Input: dimensioned drawing with shaded views. Units: mm. Origin: part minimum x, y, z. Round coordinates to 2 decimals unless told otherwise and drop trailing zeros. Loops run counter-clockwise (first coordinate to the right, second up) from the corner with the lowest first, then second, coordinate; pieces in that order, holes last.
Item 1: Section query B-B on x = 127. Return loops of the section in (y, z).
Item 2: Section query A-A on z = 101.6. Return loops of the section in (x, y).
Item 3: First-contact query: P1, Ø8, axis at x = 102, z = 48.5, coming from the -Y side; P2, Ø20.5, axis at x = 15.875, z = 57.15, coming from the -Y side. Flat tips, straight axial feed; report the tip coordinate or a pass-through.
Item 4: Section query D-D on y = 4.5. Return loops of the section in (x, z) (3 decimals), then the cut area to 3 significant figures.
Item 5: Section query C-C on z = 57.15. Return loops of the section in (x, y) (3 decimals).
Item 6: Pull-direction query (X, two-part tool) for the marked faces 1, 2 and 3; classes: released by +X, released by -X, zero draft, split by the parting line, or undercut.
Item 7: Ray query, L1, parallel to Z at x = 127, y = 3; L2, parallel to X at y = 6.25, z = 101.6; L3, parallel to X at y = 1.75, z = 57.5. Return the intervals inside material, ascending.
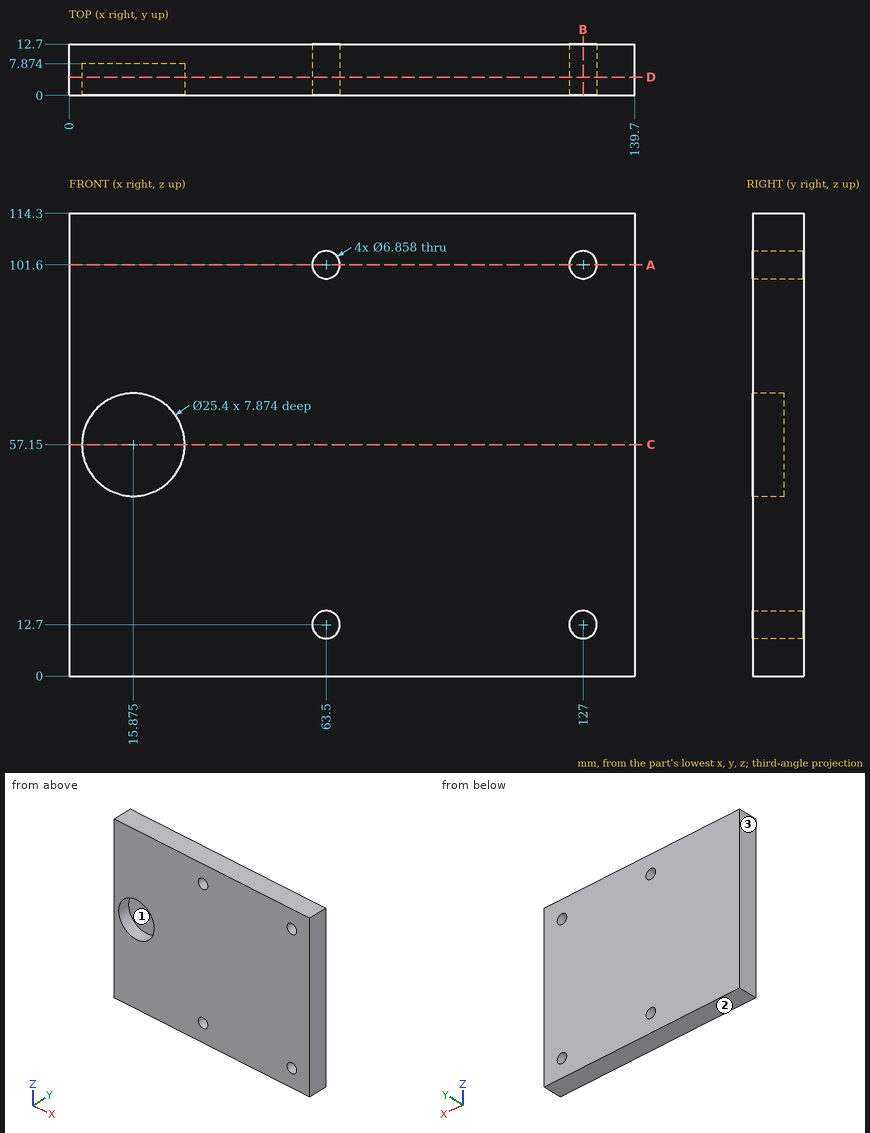
Data:
1. outline: (0, 0) - (12.7, 0) - (12.7, 9.27) - (0, 9.27) - close; (0, 16.13) - (12.7, 16.13) - (12.7, 98.17) - (0, 98.17) - close; (0, 105.03) - (12.7, 105.03) - (12.7, 114.3) - (0, 114.3) - close
2. outline: (0, 0) - (60.07, 0) - (60.07, 12.7) - (0, 12.7) - close; (66.93, 0) - (123.57, 0) - (123.57, 12.7) - (66.93, 12.7) - close; (130.43, 0) - (139.7, 0) - (139.7, 12.7) - (130.43, 12.7) - close
3. P1: stops at y = 0
3. P2: stops at y = 7.87
4. outline: (0, 0) - (139.7, 0) - (139.7, 114.3) - (0, 114.3) - close; hole circle Ø25.4 at (15.875, 57.15); hole circle Ø6.858 at (63.5, 12.7); hole circle Ø6.858 at (63.5, 101.6); hole circle Ø6.858 at (127, 12.7); hole circle Ø6.858 at (127, 101.6)
4. area: 15,300 mm2
5. outline: (0, 0) - (3.175, 0) - (3.175, 7.874) - (28.575, 7.874) - (28.575, 0) - (139.7, 0) - (139.7, 12.7) - (0, 12.7) - close
6. face 1: undercut
6. face 2: zero draft
6. face 3: released by -X
7. L1: z = 0 to 9.27, 16.13 to 98.17, 105.03 to 114.3
7. L2: x = 0 to 60.07, 66.93 to 123.57, 130.43 to 139.7
7. L3: x = 0 to 3.18, 28.57 to 139.7
